Design review of the part built by this model. Coordinates are the model's own, in mm. Face numbers are marked on the shaded views. A direction names the side the tool comes from. Give positions to 0.01 mm unless a question says otherwise; leave off trailing zeros. Order: outer loops, then holes, each group sorted by start corner. A loop starts at its lowest first (then second) coordinate and runs counter-clockwise, first axis right, second up. Notation, with made-up numbers: (6, 53) -> (38, 53) arc R16 ccw to (38, 60) -> close; hole circle Ø4 at (14, 25). An arc over 180 degrees is marked (long way). Return JSON: item names as keys, results as strings.
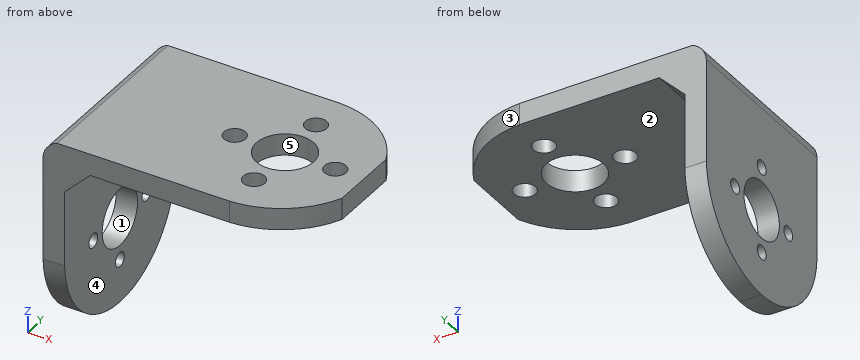
```python
from build123d import *

# Parameters (mm, degrees)
BOSS_EXTRUDE1_DEPTH = 25
CUT_EXTRUDE1_DEPTH  = 25
CUT_EXTRUDE2_DEPTH  = 25
SKETCH5_R           = 4
SKETCH5_R_2         = 1.5
CUT_EXTRUDE3_DEPTH  = 25
SKETCH6_R           = 4
SKETCH6_R_2         = 1
CUT_EXTRUDE4_DEPTH  = 25
BOSS_EXTRUDE2_DEPTH = 25


with BuildPart() as part:
    # Sketch1 → Boss-Extrude1 (new body)
    with BuildSketch(Plane(origin=(0, 0, 0), x_dir=(1, 0, 0), z_dir=(0, 1, 0))):
        with BuildLine():
            ThreePointArc((-1, 1.659075407), (-0.409273776, 0.032355851), (0.979760199, -1))
            Line((0.979760199, -1), (3.029390137, -1))
            Line((3.029390137, -1), (36, -1))
            Line((36, -1), (36, 2))
            Line((36, 2), (3.038729714, 2))
            ThreePointArc((3.038729714, 2), (3.003147911, 1.999369152), (2.967566108, 2))
            ThreePointArc((2.967566108, 2), (2.293369144, 2.293369144), (2, 2.967566108))
            Line((2, 2.967566108), (2, 28))
            Line((2, 28), (-1, 28))
            Line((-1, 28), (-1, 2))
            Line((-1, 2), (-1, 1.659075407))
        make_face()
    extrude(amount=BOSS_EXTRUDE1_DEPTH)

    # Sketch2 → Cut-Extrude1 (cut)
    with BuildSketch(Plane.ZY.offset(1)):
        with BuildLine():
            ThreePointArc((-28, 12.5), (-24.514439297, 21.163861726), (-16, 25))
            Line((-16, 25), (-28, 25))
            Line((-28, 25), (-28, 12.5))
        make_face()
        with BuildLine():
            ThreePointArc((-16, 0), (-24.514439297, 3.836138274), (-28, 12.5))
            Line((-28, 12.5), (-28, 0))
            Line((-28, 0), (-16, 0))
        make_face()
    extrude(amount=-CUT_EXTRUDE1_DEPTH, mode=Mode.SUBTRACT)

    # Sketch4 → Cut-Extrude2 (cut)
    with BuildSketch(Plane.XY.offset(1)):
        with BuildLine():
            Line((36, 25), (25, 25))
            ThreePointArc((25, 25), (31.588282141, 22.818684163), (36, 17.461413786))
            Line((36, 17.461413786), (36, 25))
        make_face()
        with BuildLine():
            Line((36, 0), (36, 7.538586214))
            ThreePointArc((36, 7.538586214), (31.588282141, 2.181315837), (25, 0))
            Line((25, 0), (36, 0))
        make_face()
    extrude(amount=-CUT_EXTRUDE2_DEPTH, mode=Mode.SUBTRACT)

    # Sketch5 → Cut-Extrude3 (cut)
    with BuildSketch(Plane.XY.offset(1)):
        with Locations((25, 12.5)):
            Circle(SKETCH5_R)
        with Locations((25, 19.5)):
            Circle(SKETCH5_R_2)
        with Locations((32, 12.5)):
            Circle(SKETCH5_R_2)
        with Locations((25, 5.5)):
            Circle(SKETCH5_R_2)
        with Locations((18, 12.5)):
            Circle(SKETCH5_R_2)
    extrude(amount=-CUT_EXTRUDE3_DEPTH, mode=Mode.SUBTRACT)

    # Sketch6 → Cut-Extrude4 (cut)
    with BuildSketch(Plane.ZY.offset(1)):
        with Locations((-16, 12.5)):
            Circle(SKETCH6_R)
        with Locations((-16, 18.5)):
            Circle(SKETCH6_R_2)
        with Locations((-10, 12.5)):
            Circle(SKETCH6_R_2)
        with Locations((-16, 6.5)):
            Circle(SKETCH6_R_2)
        with Locations((-22, 12.5)):
            Circle(SKETCH6_R_2)
    extrude(amount=-CUT_EXTRUDE4_DEPTH, mode=Mode.SUBTRACT)

    # Sketch7 → Boss-Extrude2 (add)
    with BuildSketch(Plane(origin=(0, 25, 0), x_dir=(1, 0, 0), z_dir=(0, 1, 0))):
        Polygon((0.998168154, 6.545186747), (6.456382716, 1.086972186), (0.998168154, 1.086972186), align=None)
    extrude(amount=-BOSS_EXTRUDE2_DEPTH)


solid = part.part
```
Item 1: Mouldability with a two-part tool opening along Y and no side actions: class the marked faces 3, 4 and 5 as released by +Y, released by -Y, zero draft, split by the parting line, or undercut.
Result set:
{"face 3": "released by +Y", "face 4": "zero draft", "face 5": "undercut"}
Item 2: Add section D-D (y = 4.75). Give the boundary of the cut face in (x, z).
Result set:
{"outline": "(-1, -25.31) -> (2, -25.31) -> (2, -5.54) -> (5.54, -2) -> (23.7, -2) -> (23.7, 1) -> (0.98, 1) arc R3.01 ccw to (-1, -1.66) -> close; (26.3, -2) -> (34.34, -2) -> (34.34, 1) -> (26.3, 1) -> close"}
Item 3: Add section A-A (x = 18). Give the boundary of the cut face in (y, z), plus the area to 3 significant figures.
Result set:
{"outline": "(0, -2) -> (11, -2) -> (11, 1) -> (0, 1) -> close; (14, -2) -> (25, -2) -> (25, 1) -> (14, 1) -> close", "area": "66.0 mm^2"}
Item 4: For pin 1 (5 mm diameter, centred on x = 18, y = 12.5, fed in from -Z); pin 2 (12 mm diameter, centred on y = 6, z = -25, fed in from +X), all flat-tipped, find the tip position at first contact; note any pin that passes through.
Result set:
{"pin 1": "stops at z = -2", "pin 2": "stops at x = 2"}
Item 5: Add section C-C (z = -21.5). Give the boundary of the cut face in (x, y).
Result set:
{"outline": "(-1, 1.53) -> (2, 1.53) -> (2, 11.63) -> (-1, 11.63) -> close; (-1, 13.37) -> (2, 13.37) -> (2, 23.47) -> (-1, 23.47) -> close"}
Item 6: Machinability: for the marked faces 1 and 2, which of the approach directions +Z, -Z, +X, -X, +Y, -Y give a long, thin tool a straight path to every point of the face, cutting with its end or side? Answer none if there is none.
Result set:
{"face 1": "+X, -X", "face 2": "-Z, +X, +Y, -Y"}
Item 7: Add section B-B (y = 18.5). Give the boundary of the cut face in (x, z).
Result set:
{"outline": "(-1, -26.47) -> (2, -26.47) -> (2, -17) -> (-1, -17) -> close; (-1, -15) -> (2, -15) -> (2, -5.54) -> (5.54, -2) -> (23.88, -2) -> (23.88, 1) -> (0.98, 1) arc R3.01 ccw to (-1, -1.66) -> close; (26.12, -2) -> (35.49, -2) -> (35.49, 1) -> (26.12, 1) -> close"}
Item 8: Wall thickness on L1, parallel to Y at x = 25, z = -0.9; L2, parallel to X at y = 1.75, z = -13.5; L3, parallel to Z at x = 15.5, y = 12: over which ranges is each line inside the solid? List them lowest first. Write a range as [from, to].
Result set:
{"L1": "y = [0, 4], [7, 8.5], [16.5, 18], [21, 25]", "L2": "x = [-1, 2]", "L3": "z = [-2, 1]"}
